CAD build for the part. Positions are in the model's coordinates, mm. A direction names the side the tool comes from. Round coordinates to 2 decimals unless told otherwise and drop trailing zeros. Loops run counter-clockwise (first coordinate to the right, second up) from the corner with the lowest first, then second, coordinate; pieces in that order, holes last.
from build123d import *

# Parameters (mm, degrees)
SKETCH1_W           = 10
SKETCH1_H           = 15
BOSS_EXTRUDE1_DEPTH = 85
SKETCH2_R           = 3.75
BOSS_EXTRUDE2_DEPTH = 30
FILLET2_R           = 1


with BuildPart() as part:
    # Sketch1 → Boss-Extrude1 (new, symmetric)
    with BuildSketch(Plane.XY):
        Rectangle(SKETCH1_W, SKETCH1_H)
    extrude(amount=BOSS_EXTRUDE1_DEPTH, both=True)

    # Sketch2 → Boss-Extrude2 (add)
    with BuildSketch(Plane(origin=(5, 0, 0), x_dir=(0, 0, -1), z_dir=(1, 0, 0))):
        with Locations(Location((0, 0, 0), (0, 0, 270))):
            Circle(SKETCH2_R)
    extrude(amount=BOSS_EXTRUDE2_DEPTH)

    # Fillet2
    fillet2_edges = [part.edges().sort_by_distance(p)[0] for p in [
        (-5, 7.5, 0),
        (5, 7.5, 0),
        (5, -7.5, 0),
        (-5, -7.5, 0),
    ]]
    fillet(fillet2_edges, radius=FILLET2_R)


solid = part.part
Item 1: Cut at B-B (y = 0). List the corners of the cut face in (x, z).
Verdict:
outline: (-5, -85) - (5, -85) - (5, -3.75) - (35, -3.75) - (35, 3.75) - (5, 3.75) - (5, 85) - (-5, 85) - close
Item 2: Cut at D-D (x = 19). List the corners of the cut face in (y, z), plus the area to 3 significant figures.
Verdict:
outline: circle Ø7.5 at (0, 0)
area: 44.2 mm2
Item 3: Flat gauge pins, fed straight in: P1, Ø5, axis at x = 20.5, y = 2, coming from the +Z side; P2, Ø5, axis at x = 29, y = 0, coming from the -Z side. Where does each tip first touch, or does it go through?
Verdict:
P1: stops at z = 3.75
P2: stops at z = -3.75
Item 4: 3-axis set-ups, long thin cutter, end or side, ignore diameter. For faces 1 (the flat face through (0, -7.5, 1)), 2 (the cylindrical face through (19.79, 3.746, -0.165)): which of +Z, -Z, +X, -X, +Y, -Y reach the whole face in a straight line?
Verdict:
face 1: +Z, -Z, +X, -X, -Y
face 2: +X
Item 5: Wall check: L1, parallel to X at y = 0.75, z = 34; L2, parallel to Z at x = 33, y = 0.5; L3, parallel to Z at x = 26, y = -2. Give the ranges that are in metal, low to high.
Verdict:
L1: x = -5 to 5
L2: z = -3.72 to 3.72
L3: z = -3.17 to 3.17
Item 6: Cut at C-C (z = 24). List the corners of the cut face in (x, y), plus the area to 3 significant figures.
Verdict:
outline: (-5, -6.5) arc R1 ccw to (-4, -7.5) - (4, -7.5) arc R1 ccw to (5, -6.5) - (5, 6.5) arc R1 ccw to (4, 7.5) - (-4, 7.5) arc R1 ccw to (-5, 6.5) - close
area: 149 mm2
Item 7: Cut at A-A (z = 0). List the corners of the cut face in (x, y).
Verdict:
outline: (-5, -6.5) arc R1 ccw to (-4, -7.5) - (4, -7.5) arc R1 ccw to (5, -6.5) - (5, -3.75) - (35, -3.75) - (35, 3.75) - (5, 3.75) - (5, 6.5) arc R1 ccw to (4, 7.5) - (-4, 7.5) arc R1 ccw to (-5, 6.5) - close
